```python
from build123d import *

# Parameters (mm, degrees)
BOSS_EXTRUDE1_DEPTH = 43.5102


with BuildPart() as part:
    # Sketch2 → Boss-Extrude1 (new body)
    with BuildSketch(Plane.XY):
        with BuildLine():
            Line((-4.366026501, 25.941944541), (-1.27, 34.448207442))
            ThreePointArc((-1.27, 34.448207442), (0, 34.47161), (1.27, 34.448207442))
            Line((1.27, 34.448207442), (4.366026501, 25.941944541))
            ThreePointArc((4.366026501, 25.941944541), (4.83385814, 25.858857079), (5.300112805, 25.767333549))
            Line((5.300112805, 25.767333549), (11.259888122, 32.580773709))
            ThreePointArc((11.259888122, 32.580773709), (12.452581833, 32.143819028), (13.628367585, 31.663219877))
            Line((13.628367585, 31.663219877), (13.442509735, 22.612952173))
            ThreePointArc((13.442509735, 22.612952173), (13.848735094, 22.366475142), (14.250442508, 22.11270138))
            Line((14.250442508, 22.11270138), (22.26906596, 26.31312595))
            ThreePointArc((22.26906596, 26.31312595), (23.223373486, 25.474827181), (24.14614861, 24.601939015))
            Line((24.14614861, 24.601939015), (20.703507542, 16.229955312))
            ThreePointArc((20.703507542, 16.229955312), (20.993263634, 15.8533768), (21.276170986, 15.471626358))
            Line((21.276170986, 15.471626358), (30.270683044, 16.491744725))
            ThreePointArc((30.270683044, 16.491744725), (30.857719866, 15.365318762), (31.402858467, 14.218029965))
            Line((31.402858467, 14.218029965), (25.168381933, 7.655013053))
            ThreePointArc((25.168381933, 7.655013053), (25.302535593, 7.199192074), (25.428434676, 6.741022466))
            Line((25.428434676, 6.741022466), (34.184076646, 4.443061991))
            ThreePointArc((34.184076646, 4.443061991), (34.324560189, 3.180638903), (34.418438279, 1.913897183))
            Line((34.418438279, 1.913897183), (26.234126882, -1.953781138))
            ThreePointArc((26.234126882, -1.953781138), (26.194559914, -2.427283433), (26.14644736, -2.899993864))
            Line((26.14644736, -2.899993864), (33.480721277, -8.205680884))
            ThreePointArc((33.480721277, -8.205680884), (33.155678459, -9.433603865), (32.785617282, -10.648718018))
            Line((32.785617282, -10.648718018), (23.756807626, -11.298706359))
            ThreePointArc((23.756807626, -11.298706359), (23.54886377, -11.725940863), (23.333237446, -12.149349953))
            Line((23.333237446, -12.149349953), (28.255608976, -19.746201087))
            ThreePointArc((28.255608976, -19.746201087), (27.508938632, -20.773786158), (26.724917, -21.773164845))
            Line((26.724917, -21.773164845), (18.07099986, -19.117678678))
            ThreePointArc((18.07099986, -19.117678678), (17.722763084, -19.440945003), (17.36874452, -19.757869009))
            Line((17.36874452, -19.757869009), (19.214420114, -28.619887416))
            ThreePointArc((19.214420114, -28.619887416), (18.14696421, -29.308353518), (17.054868589, -29.95702511))
            Line((17.054868589, -29.95702511), (9.944603428, -24.354702557))
            ThreePointArc((9.944603428, -24.354702557), (9.503105039, -24.530341795), (9.058506404, -24.697978373))
            Line((9.058506404, -24.697978373), (7.578217344, -33.628299361))
            ThreePointArc((7.578217344, -33.628299361), (6.334141716, -33.884665333), (5.081465671, -34.095023136))
            Line((5.081465671, -34.095023136), (0.475133198, -26.302488901))
            ThreePointArc((0.475133198, -26.302488901), (0, -26.30678), (-0.475133198, -26.302488901))
            Line((-0.475133198, -26.302488901), (-5.081465671, -34.095023136))
            ThreePointArc((-5.081465671, -34.095023136), (-6.334141716, -33.884665333), (-7.578217344, -33.628299361))
            Line((-7.578217344, -33.628299361), (-9.058506404, -24.697978373))
            ThreePointArc((-9.058506404, -24.697978373), (-9.503105039, -24.530341795), (-9.944603428, -24.354702557))
            Line((-9.944603428, -24.354702557), (-17.054868589, -29.95702511))
            ThreePointArc((-17.054868589, -29.95702511), (-18.14696421, -29.308353518), (-19.214420114, -28.619887416))
            Line((-19.214420114, -28.619887416), (-17.36874452, -19.757869009))
            ThreePointArc((-17.36874452, -19.757869009), (-17.722763084, -19.440945003), (-18.07099986, -19.117678678))
            Line((-18.07099986, -19.117678678), (-26.724917, -21.773164845))
            ThreePointArc((-26.724917, -21.773164845), (-27.508938632, -20.773786158), (-28.255608976, -19.746201087))
            Line((-28.255608976, -19.746201087), (-23.333237446, -12.149349953))
            ThreePointArc((-23.333237446, -12.149349953), (-23.54886377, -11.725940863), (-23.756807626, -11.298706359))
            Line((-23.756807626, -11.298706359), (-32.785617282, -10.648718018))
            ThreePointArc((-32.785617282, -10.648718018), (-33.155678459, -9.433603865), (-33.480721277, -8.205680884))
            Line((-33.480721277, -8.205680884), (-26.14644736, -2.899993864))
            ThreePointArc((-26.14644736, -2.899993864), (-26.194559914, -2.427283433), (-26.234126882, -1.953781138))
            Line((-26.234126882, -1.953781138), (-34.418438279, 1.913897183))
            ThreePointArc((-34.418438279, 1.913897183), (-34.324560189, 3.180638903), (-34.184076646, 4.443061991))
            Line((-34.184076646, 4.443061991), (-25.428434676, 6.741022466))
            ThreePointArc((-25.428434676, 6.741022466), (-25.302535593, 7.199192074), (-25.168381933, 7.655013053))
            Line((-25.168381933, 7.655013053), (-31.402858467, 14.218029965))
            ThreePointArc((-31.402858467, 14.218029965), (-30.857719866, 15.365318762), (-30.270683044, 16.491744725))
            Line((-30.270683044, 16.491744725), (-21.276170986, 15.471626358))
            ThreePointArc((-21.276170986, 15.471626358), (-20.993263634, 15.8533768), (-20.703507542, 16.229955312))
            Line((-20.703507542, 16.229955312), (-24.14614861, 24.601939015))
            ThreePointArc((-24.14614861, 24.601939015), (-23.223373486, 25.474827181), (-22.26906596, 26.31312595))
            Line((-22.26906596, 26.31312595), (-14.250442508, 22.11270138))
            ThreePointArc((-14.250442508, 22.11270138), (-13.848735094, 22.366475142), (-13.442509735, 22.612952173))
            Line((-13.442509735, 22.612952173), (-13.628367585, 31.663219877))
            ThreePointArc((-13.628367585, 31.663219877), (-12.452581833, 32.143819028), (-11.259888122, 32.580773709))
            Line((-11.259888122, 32.580773709), (-5.300112805, 25.767333549))
            ThreePointArc((-5.300112805, 25.767333549), (-4.83385814, 25.858857079), (-4.366026501, 25.941944541))
        make_face()
    extrude(amount=BOSS_EXTRUDE1_DEPTH)


solid = part.part
```
Design review of the part built by this model. Coordinates are the model's own, in mm. A direction names the side the tool comes from. Round coordinates to 2 decimals unless told otherwise and drop trailing zeros. Order: outer loops, then holes, each group sorted by start corner. A loop starts at its lowest first (then second) coordinate and runs counter-clockwise, first axis right, second up. Notation, with made-up numbers: M 48,-27 L 64,-27 A35 cw 64,11 Z; hole C 7.5,-31 d5. An arc over 180 degrees is marked long. Put each result on its own line as item: value.
Q1. Insertion check: pin 1 Ø12 at (y, z) = (16.5, 6.5) entering from +X; pin 2 Ø10 at (x, y) = (15, 19) entering from -Z; pin 3 Ø4 at (x, z) = (13.5, 13.5) entering from +Y; pin 4 Ø4 at (y, z) = (19.5, 25) entering from +X. Each pin has a flat end and moves straight along its axis. Give the tip position at first contact, or say it passes through.
Reported:
pin 1: x = 31.4
pin 2: z = 0
pin 3: y = 32.5
pin 4: x = 22.87
Q2. Draft analysis for pull direction Y (two halves, no side actions). For faces 1 (the face through (-13.45, -27.117, 21.451)), 2 (the face through (-18.316, 24.242, 21.451)), 3 (the face through (28.33, -10.97, 21.45)), state which applies: released by +Y, released by -Y, zero draft, split by the parting line, or undercut.
Reported:
face 1: released by -Y
face 2: released by +Y
face 3: undercut
Q3. Machinability: for faces 4 (the face through (-25.84, 15.99, 21.45)), 5 (the face through (-29.868, 5.576, 21.451)), 6 (the face through (18.2, 24.18, 21.45)), which of the approach directions +Z, -Z, +X, -X, +Y, -Y give a long, thin tool a straight path to every point of the face, cutting with its end or side? Answer none if there is none.
Reported:
face 4: +Z, -Z
face 5: +Z, -Z, -X
face 6: +Z, -Z, +Y
Q4. To check wall thickness, follow line 1 (X direction, y = 25.5, z = 19.5); line 2 (X direction, y = -27, z = 26.5); line 3 (Y direction, x = 30.5, z = 36). State the ranges of each line that lie inside material, in increasing order.
Reported:
line 1: -23.2 to -20.72, -13.5 to 13.5, 20.72 to 23.2
line 2: -18.88 to -13.3, -8.68 to -0.89, 0.89 to 8.68, 13.3 to 18.88
line 3: -10.81 to -6.05, 0.06 to 5.41, 13.27 to 16.06
Q5. Consider section A-A (y = -7). State the section outline as (x, z) points, and give its area (3 significant figures).
Reported:
outline: M -31.81,0 L 31.81,0 L 31.81,43.51 L -31.81,43.51 Z
area: 2,770 mm²
